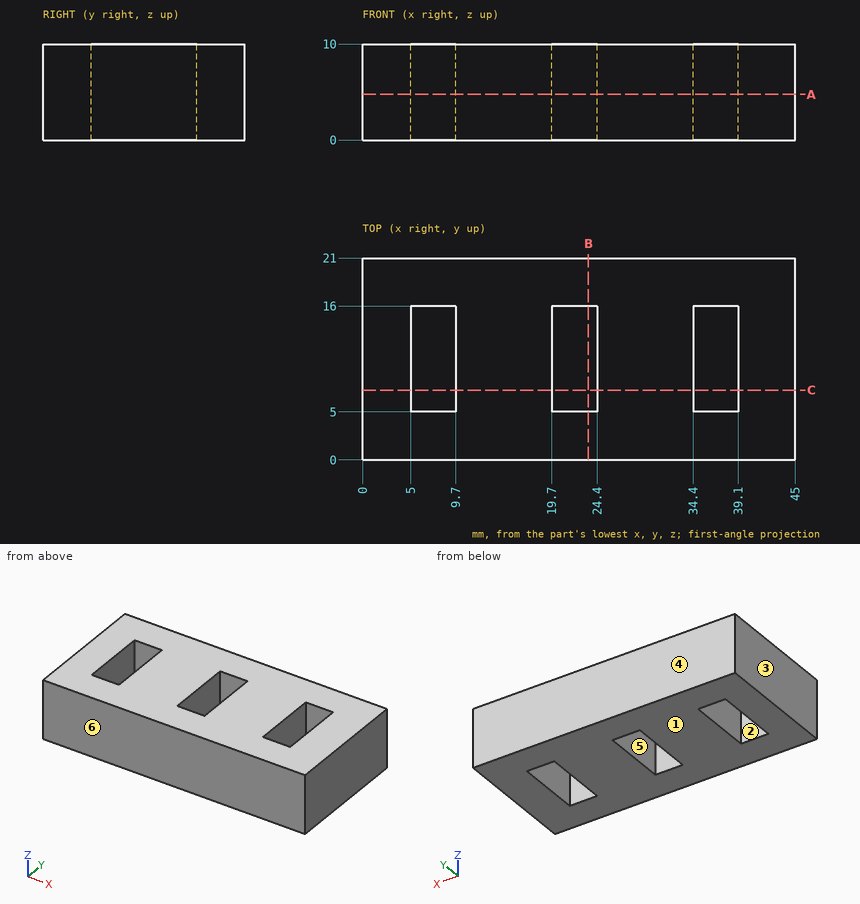
Part print with two shaded views. Sizes in mm from the minimum x, y, z corner. A direction names the side the tool comes from. Round coordinates to 2 decimals unless told otherwise and drop trailing zeros. Order: outer loops, then holes, each group sorted by start corner. A loop starts at its lowest first (then second) coordinate and runs counter-clockwise, first axis right, second up. Notation, with made-up numbers: (42.25, 67) -> (51.25, 67) arc R15 ccw to (51.25, 75) -> close; hole circle Ø1 at (17, 75.5). An arc over 180 degrees is marked (long way). Use one line per item in the form item = value.
Item 1: Cut at B-B, the plane x = 23.5. Write the cut outline in (y, z).
Returned:
outline = (0, 0) -> (5, 0) -> (5, 10) -> (0, 10) -> close; (16, 0) -> (21, 0) -> (21, 10) -> (16, 10) -> close
Item 2: Drill centre lines: line 1 (X direction, y = 12.5, z = 1.5); line 2 (Y direction, x = 36, z = 9.5). Where is each one in solid material? Low to high.
Returned:
line_1 = 0 to 5, 9.7 to 19.7, 24.4 to 34.4, 39.1 to 45
line_2 = 0 to 5, 16 to 21
Item 3: Tool access for the marked faces 1 and 2: list every direction of +Z, -Z, +X, -X, +Y, -Y with a clear straight run to the whole face (end or side of a thin tool).
Returned:
face_1 = -Z, +X, -X, +Y, -Y
face_2 = +Z, -Z
Item 4: Cut at C-C, the plane y = 7.25. Write the cut outline in (x, z).
Returned:
outline = (0, 0) -> (5, 0) -> (5, 10) -> (0, 10) -> close; (9.7, 0) -> (19.7, 0) -> (19.7, 10) -> (9.7, 10) -> close; (24.4, 0) -> (34.4, 0) -> (34.4, 10) -> (24.4, 10) -> close; (39.1, 0) -> (45, 0) -> (45, 10) -> (39.1, 10) -> close
Item 5: Cut at A-A, the plane z = 4.75. Write the cut outline in (x, y).
Returned:
outline = (0, 0) -> (45, 0) -> (45, 21) -> (0, 21) -> close; hole (5, 5) -> (9.7, 5) -> (9.7, 16) -> (5, 16) -> close; hole (19.7, 5) -> (24.4, 5) -> (24.4, 16) -> (19.7, 16) -> close; hole (34.4, 5) -> (39.1, 5) -> (39.1, 16) -> (34.4, 16) -> close
Item 6: Pull direction Y, two halves, no side cores. Call the marked faces 3, 4, 5 and 6: released by +Y, released by -Y, zero draft, split by the parting line, or undercut.
Returned:
face_3 = zero draft
face_4 = released by +Y
face_5 = undercut
face_6 = released by -Y
